```python
from build123d import *

# Parameters (mm, degrees)
CROQUIS1_W                  = 170
CROQUIS1_H                  = 50
SALIENTE_EXTRUIR1_DEPTH     = 4
SALIENTE_EXTRUIR2_DEPTH     = 100
SALIENTE_EXTRUIR3_DEPTH     = 25
SALIENTE_EXTRUIR4_DEPTH     = 64
SALIENTE_EXTRUIR5_DEPTH     = 25
CROQUIS9_W                  = 17
CROQUIS9_H                  = 17.5
CROQUIS9_W_2                = 56
CORTAR_EXTRUIR1_DEPTH       = 100
CROQUIS11_W                 = 64
CROQUIS11_H                 = 85
CORTAR_EXTRUIR4_DEPTH       = 15
CROQUIS12_R                 = 1.75
CORTAR_EXTRUIR5_DEPTH       = 15
CORTAR_EXTRUIR6_DEPTH       = 1
CROQUIS16_W                 = 170
CROQUIS16_H                 = 3.747948586
CORTAR_EXTRUIR7_DEPTH       = 100
CORTAR_EXTRUIR10_DEPTH      = 139.192800102
CORTAR_EXTRUIR10_DEPTH_BACK = 139.192800102
CROQUIS20_R                 = 1.25
CROQUIS21_W                 = 5.666666666
CROQUIS21_H                 = 96.899748192
CORTAR_EXTRUIR11_DEPTH      = 10


with BuildPart() as part:
    # Croquis1 → Saliente-Extruir1 (new body)
    with BuildSketch(Plane.XY):
        Rectangle(CROQUIS1_W, CROQUIS1_H)
    extrude(amount=SALIENTE_EXTRUIR1_DEPTH)

    # Croquis3 → Saliente-Extruir2 (add)
    with BuildSketch(Plane.XY.offset(4)):
        Polygon((-85, 7.5), (85, 7.5), (85, -7.5), (60, -7.5), (60, -11.921199344), (56, -11.921199344), (54.5, -11.921199344), (54.5, -8.921199344), (56, -8.921199344), (56, -2.921199344), (36, -2.921199344), (36, -8.921199344), (37.5, -8.921199344), (37.5, -11.921199344), (36, -11.921199344), (32, -11.921199344), (32, -7.5), (-32, -7.5), (-32, -11.921199344), (-36, -11.921199344), (-37.5, -11.921199344), (-37.5, -8.921199344), (-36, -8.921199344), (-36, -2.921199344), (-56, -2.921199344), (-56, -8.921199344), (-54.5, -8.921199344), (-54.5, -11.921199344), (-56, -11.921199344), (-60, -11.921199344), (-60, -7.5), (-85, -7.5), align=None)
    extrude(amount=SALIENTE_EXTRUIR2_DEPTH)

    # Croquis4 → Saliente-Extruir3 (add)
    with BuildSketch(Plane.ZY.offset(85)):
        Polygon((4, -25), (19, -7.5), (4, -7.5), align=None)
    extrude(amount=-SALIENTE_EXTRUIR3_DEPTH)

    # Croquis5 → Saliente-Extruir4 (add)
    with BuildSketch(Plane.ZY.offset(-32)):
        Polygon((19, -7.5), (4, -25), (4, -7.5), align=None)
    extrude(amount=SALIENTE_EXTRUIR4_DEPTH)

    # Croquis7 → Saliente-Extruir5 (add)
    with BuildSketch(Plane(origin=(60, 0, 0), x_dir=(0, 0, -1), z_dir=(1, 0, 0))):
        Polygon((-4, -25), (-19, -7.5), (-4, -7.5), align=None)
    extrude(amount=SALIENTE_EXTRUIR5_DEPTH)

    # Croquis9 → Cortar-Extruir1 (cut)
    with BuildSketch(Plane.XY.offset(104)):
        with Locations((-72.5, -16.25)):
            Rectangle(CROQUIS9_W, CROQUIS9_H)
        with Locations((0, -16.25)):
            Rectangle(CROQUIS9_W_2, CROQUIS9_H)
        with Locations((72.5, -16.25)):
            Rectangle(CROQUIS9_W, CROQUIS9_H)
    extrude(amount=-CORTAR_EXTRUIR1_DEPTH, mode=Mode.SUBTRACT)

    # Croquis11 → Cortar-Extruir4 (cut)
    with BuildSketch(Plane.XZ.offset(7.5)):
        with Locations((0, 61.5)):
            Rectangle(CROQUIS11_W, CROQUIS11_H)
    extrude(amount=-CORTAR_EXTRUIR4_DEPTH, mode=Mode.SUBTRACT)

    # Croquis12 → Cortar-Extruir5 (cut)
    with BuildSketch(Plane.XY.offset(4)):
        with Locations((-72.5, 15.138462845)):
            Circle(CROQUIS12_R)
        with Locations((-72.5, -15.138462845)):
            Circle(CROQUIS12_R)
        with Locations((72.5, -15.138462845)):
            Circle(CROQUIS12_R)
        with Locations((72.5, 15.138462845)):
            Circle(CROQUIS12_R)
    extrude(amount=-CORTAR_EXTRUIR5_DEPTH, mode=Mode.SUBTRACT)

    # Croquis14 → Cortar-Extruir6 (cut)
    with BuildSketch(Plane.ZY.offset(85)):
        Polygon((19, -7.5), (4, -7.5), (4, -25), align=None)
    extrude(amount=-CORTAR_EXTRUIR6_DEPTH, mode=Mode.SUBTRACT)

    # Croquis16 → Cortar-Extruir7 (cut)
    with BuildSketch(Plane.XY.offset(104)):
        with Locations((0, 5.626025707)):
            Rectangle(CROQUIS16_W, CROQUIS16_H)
    extrude(amount=-CORTAR_EXTRUIR7_DEPTH, mode=Mode.SUBTRACT)

    # Croquis20 → Cortar-Extruir10 (cut, two sides: drawn at the far end of the back side and taken through both)
    with BuildSketch(Plane.XZ.offset(7.5).offset(-CORTAR_EXTRUIR10_DEPTH_BACK)):
        with Locations(Location((-78.5, 86.5, 0), (0, 0, 270))):
            Circle(CROQUIS20_R)
        with Locations(Location((-66.5, 86.5, 0), (0, 0, 270))):
            Circle(CROQUIS20_R)
        with Locations(Location((-66.5, 36.5, 0), (0, 0, 270))):
            Circle(CROQUIS20_R)
        with Locations(Location((-78.5, 36.5, 0), (0, 0, 270))):
            Circle(CROQUIS20_R)
        with Locations(Location((66.5, 36.5, 0), (0, 0, 270))):
            Circle(CROQUIS20_R)
        with Locations(Location((78.5, 36.5, 0), (0, 0, 270))):
            Circle(CROQUIS20_R)
        with Locations(Location((66.5, 86.5, 0), (0, 0, 270))):
            Circle(CROQUIS20_R)
        with Locations(Location((78.5, 86.5, 0), (0, 0, 270))):
            Circle(CROQUIS20_R)
    extrude(amount=CORTAR_EXTRUIR10_DEPTH + CORTAR_EXTRUIR10_DEPTH_BACK, mode=Mode.SUBTRACT)

    # Croquis21 → Cortar-Extruir11 (cut)
    with BuildSketch(Plane.XZ.offset(2.921199344)):
        with Locations((-46, 55.550125904)):
            Rectangle(CROQUIS21_W, CROQUIS21_H)
        with Locations((46, 55.550125904)):
            Rectangle(CROQUIS21_W, CROQUIS21_H)
    extrude(amount=-CORTAR_EXTRUIR11_DEPTH, mode=Mode.SUBTRACT)


solid = part.part
```
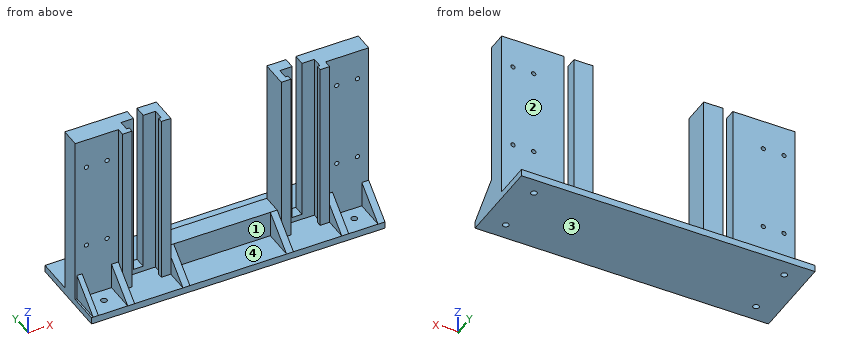
Verification items for the finished model (mm, model axes). Face numbers are marked on the shaded views. A direction names the side the tool comes from. Coordinates: 2 decimals unless noted, no trailing zeros. Loops run counter-clockwise (first coordinate to the right, second up) from the corner with the lowest first, then second, coordinate; pieces in that order, holes last. Notation, with made-up numbers: (35, 36) -> (61, 36) arc R24 ccw to (61, 69) -> close; hole circle Ø11 at (26.25, -10.5). An arc over 180 degrees is marked (long way). Put each result on its own line as item: value.
1. Section check C-C, the plane z = 46. Give the number of separate pieces and of enclosed holes in the cut face, then the cut area to 3 significant figures.
Result set:
separate pieces: 4
enclosed holes: 0
area: 1,020 mm^2
2. Section check A-A, the plane x = -72.5. Record the boundary of the cut face in (y, z).
Result set:
outline: (-25, 0) -> (-16.89, 0) -> (-16.89, 4) -> (-25, 4) -> close; (-13.39, 0) -> (13.39, 0) -> (13.39, 4) -> (3.75, 4) -> (3.75, 104) -> (-7.5, 104) -> (-7.5, 4) -> (-13.39, 4) -> close; (16.89, 0) -> (25, 0) -> (25, 4) -> (16.89, 4) -> close
3. Section check D-D, the plane y = 10. Record the boundary of the cut face in (x, z).
Result set:
outline: (-85, 0) -> (85, 0) -> (85, 4) -> (-85, 4) -> close
4. Section check B-B, the plane x = 45.5. Record the boundary of the cut face in (y, z), then the cut area to 3 significant figures.
Result set:
outline: (-25, 0) -> (25, 0) -> (25, 4) -> (3.75, 4) -> (3.75, 7.1) -> (-2.92, 7.1) -> (-2.92, 4) -> (-25, 4) -> close
area: 221 mm^2
5. Mould release check, pull along X, two halves, no side actions. Record for the marked faces 1 and 2: pulls with the +X half, pulls with the -X half, needs draft (parallel to the pull), parting line crosses it, or undercut.
Result set:
face 1: undercut
face 2: needs draft
6. Tool access check on the marked faces 3 and 4. Record the directions out of +Z, -Z, +X, -X, +Y, -Y that give a thin tool (end or side, any length) a straight path to the whole face; none if there is none.
Result set:
face 3: -Z, +X, -X, +Y, -Y
face 4: +Z, -Y
7. Gauge pin test, flat ends, axial feed: P1, Ø4.5, axis at x = -46.5, y = 1, coming from the +Z side; P2, Ø16.5, axis at y = -17, z = 13.5, coming from the -X side; P3, Ø3, axis at x = -32.5, y = -12, coming from the +Z side; P4, Ø5, axis at x = 76, y = -19, coming from the +Z side. Record the tip position at first contact, or that the pin passes through.
Result set:
P1: stops at z = 7.1
P2: stops at x = -84
P3: stops at z = 104
P4: stops at z = 4
8. Thickness scan on line 1 (Z direction, x = -78.5, y = -1.5); line 2 (Z direction, x = 66, y = 0); line 3 (Y direction, x = 72.5, z = 2.3). Record the ranges inside material, lowest first.
Result set:
line 1: z = 0 to 35.25, 37.75 to 85.25, 87.75 to 104
line 2: z = 0 to 35.35, 37.65 to 85.35, 87.65 to 104
line 3: y = -25 to -16.89, -13.39 to 13.39, 16.89 to 25
